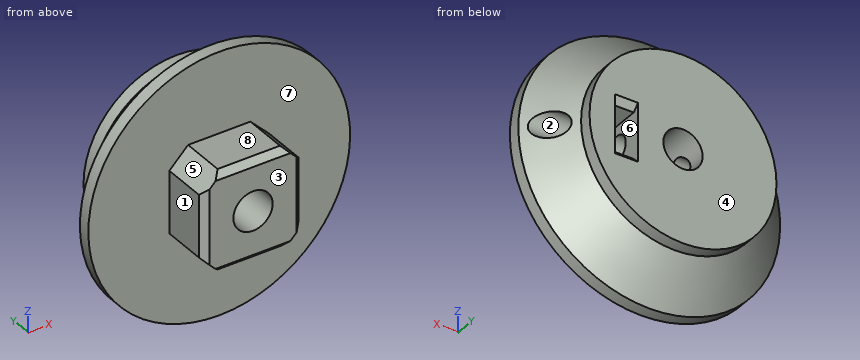
Autodesk Inventor part; units mm, degrees
ref_plane "YZ Plane" through (0, 0, 0) normal (1, 0, 0) x (0, 1, 0)
ref_plane "XZ Plane" through (0, 0, 0) normal (0, 1, 0) x (-1, 0, 0)
ref_plane "XY Plane" through (0, 0, 0) normal (0, 0, 1) x (1, 0, 0)
sketch "Boceto1" plane through (0, 0, 0) normal (0, 1, 0) x (-1, 0, 0)
  circle A0 centre (0, 0) radius 3.15
  circle A1 centre (0, 0) radius 15
  line L0 (-7.225, 3.7) -> (-10.925, 3.7)
  line L1 (-10.925, 3.7) -> (-10.925, -3.7)
  line L2 (-10.925, -3.7) -> (-7.225, -3.7)
  line L3 (-7.225, -3.7) -> (-7.225, 3.7)
  circle A2 centre (0, 0) radius 9.8003 construction
  line L4 (6.8168, -4.407) -> (0.4082, -8.107)
  line L5 (8.6668, -7.6113) -> (6.8168, -4.407)
  line L6 (2.2582, -11.3113) -> (8.6668, -7.6113)
  line L7 (0.4082, -8.107) -> (2.2582, -11.3113)
  line L8 (0.4082, 8.107) -> (6.8168, 4.407)
  line L9 (2.2582, 11.3113) -> (0.4082, 8.107)
  line L10 (8.6668, 7.6113) -> (2.2582, 11.3113)
  line L11 (6.8168, 4.407) -> (8.6668, 7.6113)
  point P0 (-7.225, 0)
  point P1 (-9.075, 3.7)
  point P2 (3.6125, -6.257)
  point P3 (1.3332, -9.7092)
  point P4 (3.6125, 6.257)
  point P5 (7.7418, 6.0092)
  dimension "d0" = 6.3
  dimension "tuerca" = 7.4
  dimension "d2" = 11.85
  dimension "d3" = 6.6503
  dimension "d4" = 3.7
  dimension "d18" = 360
  dimension "d26" = 30
  dimension "d27" = 4.075
  dimension "d28" = 4.075
extrude "Extrusión1" add sketch "Boceto1" along normal blind 10 contours A1 | L5 L6 L7 L4 | L9 L10 L11 L8
sketch "Boceto4" plane through (0, 0, 0) normal (1, 0, 0) x (0, 1, 0)
  line L0 (0, -15) -> (10, -15)
  line L1 (0, -15) -> (0, -21)
  line L2 (0, -21) -> (2, -21)
  line L3 (2, -21) -> (8, -15)
  line L4 (0, 0) -> (7.4976, 0)
  dimension "d47" = 45
  dimension "d48" = 21
  dimension "d49" = 2
revolve "Revolución1" add sketch "Boceto4" angle 360 about axis through (0, 0, 0) along (0, 1, 0)
sketch "Boceto2" plane through (7.225, 0, -3.7) normal (1, 0, 0) x (0, 0, -1)
  line L0 (0, 0) -> (-7.4, 0)
  line L1 (0, 0) -> (0, 10) construction
  line L2 (-7.4, 10) -> (0, 10) construction
  line L3 (-7.4, 0) -> (-7.4, 10) construction
  line L4 (-7.4, 0) -> (0, 10) construction
  circle A0 centre (-3.7, 5) radius 2.1
  line L5 (0, 2.6329) -> (-4.5603, 0)
  line L6 (-2.8397, 0) -> (-7.4, 2.6329)
  line L7 (-7.4, 2.6329) -> (-7.4, 0)
  line L8 (0, 2.6329) -> (0, 0)
  point P0 (-3.7, 0)
  dimension "d7" = 4.2
  dimension "d8" = 120
  dimension "d9" = 3.9
extrude "Extrusión2" cut sketch "Boceto2" along normal mid plane 30 contours A0
extrude "Extrusión3" add sketch "Boceto2" along normal up to next contours L0 L6 L5 L8 | L0 L5 L6 | L0 L7 L6 L5
sketch "Boceto3" plane through (0, 0, 0) normal (0, -1, 0) x (1, 0, 0)
  circle A0 centre (0, 0) radius 3.15
  circle A1 centre (0, 0) radius 27.5
  line L0 (-5, 8) -> (5, 8)
  line L1 (8, 5) -> (8, -5)
  line L2 (5, -8) -> (-5, -8)
  line L3 (-8, -5) -> (-8, 5)
  line L4 (-8, 5) -> (-5, 8)
  line L5 (5, 8) -> (8, 5)
  line L6 (8, -5) -> (5, -8)
  line L7 (-8, -5) -> (-5, -8)
  point P0 (-8, 8)
  point P1 (8, -8)
  point P2 (8, 8)
  point P3 (-8, -8)
  point P4 (-8, 0)
  point P5 (0, -8)
  dimension "d32" = 16
  dimension "d33" = 55
  dimension "d39" = 3
  dimension "d40" = 3
  dimension "d41" = 3
  dimension "d42" = 3
  dimension "d43" = 3
  dimension "d44" = 3
  dimension "d45" = 3
  dimension "d46" = 3
extrude "Extrusión4" add sketch "Boceto3" along normal blind 8 contours L0 L5 L1 L6 L2 L7 L3 L4
chamfer "Chaflán1" distance 1 angle 45 2 edges at (9.075, 10, 3.7) (9.075, 10, -3.7)
chamfer "Chaflán3" distance 1 angle 45 4 edges at (0, -8, 8) (-8, -8, 0) (0, -8, -8) (8, -8, 0)
equation "\"d28\" = d27"
properties part number "dado polea correa motor"
Here's how the part is built. I have some questions about the finished solid (model axes, mm). Face numbers are marked on the shaded views. A direction names the side the tool comes from. Coordinates: 2 decimals unless noted, no trailing zeros. Order: outer loops, then holes, each group sorted by start corner. A loop starts at its lowest first (then second) coordinate and runs counter-clockwise, first axis right, second up. Notation, with made-up numbers: (41.5, 1) - (70.5, 1) arc R28 ccw to (70.5, 34) - close; hole circle Ø10 at (40.5, 56.5). An arc over 180 degrees is marked (long way). One line per question, with ' | ' between items. Start each with the question number.
1. If we mould it in two halves opening along Y, with no side actions, what happens to the marked faces 1, 2 and 3? For each: released by +Y, released by -Y, zero draft, split by the parting line, or undercut.
2. If we section it at A-A (x = 0): Write out the boundary of the cut face in (y, z).
3. Which directions (+Z, -Z, +X, -X, +Y, -Y) give clear straight access to the entire face, cutting with the end or side of a thin tool? Please do the marked faces 4, 5, 6, 7 and 8.
4. Please list where these lines run through material, in increasing order: line 1 along X through (y, z) = (8.75, 0) (3 decimals); line 2 along X through (y, z) = (3.75, 2) (3 decimals); line 3 along Z through (x, y) = (0, -3.75). Write a range as [from, to].
5. I'm going to push flat-ended pins straight in: pin 1 Ø6 at (x, z) = (10.5, -0.5) entering from +Y; pin 2 Ø3.5 at (y, z) = (5, 0) entering from +X (3 decimals); pin 3 Ø4 at (x, z) = (0, 0) entering from +Y; pin 4 Ø1 at (x, z) = (-16.5, -5.5) entering from -Y. Where does each tip first touch, or does it pass through?
6. If we section it at D-D (y = 5): Write out the boundary of the cut face in (x, z) (3 decimals).
7. If we section it at B-B (y = -1.25): Write out the boundary of the cut face in (x, z), and give its area (3 significant figures).
8. If we section it at C-C (z = -1): Give the number of separate pieces and of enclosed holes in the cut face, and give its area (3 significant figures).
Model answer:
1) face 1: zero draft | face 2: undercut | face 3: released by -Y
2) outline: (-8, -7) - (-7, -8) - (0, -8) - (0, -21) - (2, -21) - (8, -15) - (10, -15) - (10, -3.15) - (-8, -3.15) - close; (-8, 3.15) - (10, 3.15) - (10, 15) - (8, 15) - (2, 21) - (0, 21) - (0, 8) - (-7, 8) - (-8, 7) - close
3) face 4: +Z, -Z, +X, -X, +Y | face 5: +Z, -X, -Y | face 6: +Y | face 7: -Y | face 8: +Z, +X, -X, -Y
4) line 1: x = [-15, -3.15], [3.15, 7.225], [10.925, 15] | line 2: x = [-19.146, -2.434], [2.434, 7.225], [10.925, 19.146] | line 3: z = [-8, -3.15], [3.15, 8]
5) pin 1: stops at y = 10 | pin 2: stops at x = -7.775 | pin 3: passes through | pin 4: stops at y = 0
6) outline: (-7.775, -2.1) - (-7.775, 2.1) - (-2.348, 2.1) arc R3.15 cw to (2.348, 2.1) - (7.225, 2.1) - (7.225, 3.7) - (10.925, 3.7) - (10.925, 2.1) - (17.877, 2.1) arc R18 ccw (long way) to (17.877, -2.1) - (10.925, -2.1) - (10.925, -3.7) - (7.225, -3.7) - (7.225, -2.1) - (2.348, -2.1) arc R3.15 cw to (-2.348, -2.1) - close
7) outline: (-8, -5) - (-5, -8) - (5, -8) - (8, -5) - (8, 5) - (5, 8) - (-5, 8) - (-8, 5) - close; hole circle Ø6.3 at (0, 0) | area: 207 mm²
8) separate pieces: 4 | enclosed holes: 0 | area: 287 mm²
